from build123d import *

# Parameters (mm, degrees)
BOSS_EXTRUDE1_DEPTH = 5
SKETCH2_R           = 4
CUT_EXTRUDE1_DEPTH  = 5


with BuildPart() as part:
    # Sketch1 → Boss-Extrude1 (new body)
    with BuildSketch(Plane.XY):
        Polygon((-27.36941191, 43.029850731), (-27.36941191, -10.970149254), (-72.36941191, -10.970149254), (-142.36941191, -10.970149254), (-59.112279179, 4.938410019), align=None)
    extrude(amount=BOSS_EXTRUDE1_DEPTH)

    # Sketch2 → Cut-Extrude1 (cut)
    with BuildSketch(Plane.XY.offset(5)):
        with Locations((-37.419438967, -3.470149254)):
            Circle(SKETCH2_R)
        with Locations((-37.419438967, 11.529850746)):
            Circle(SKETCH2_R)
        with Locations((-52.419438967, -4.105668706)):
            Circle(SKETCH2_R)
    extrude(amount=-CUT_EXTRUDE1_DEPTH, mode=Mode.SUBTRACT)


solid = part.part
CAD build for the part. Positions are in the model's coordinates, mm. Coordinates: 2 decimals unless noted, no trailing zeros. Write each loop counter-clockwise with the first axis right and the second up, starting at its lowest first coordinate (ties: lowest second). Pieces come first, ordered by that corner, then holes. Notation, with made-up numbers: (87, 36) - (129, 36) arc R14 cw to (129, 62) - close; hole circle Ø5 at (61.5, 13.5). An arc over 180 degrees is marked (long way). Use a Markdown table: item, result. Add a question column.
Item 1: Band-saw the part on C-C, the plane z = 3.7. Give the cut face in (x, y), and give its area (3 significant figures).
Item 2: Mould opens along X. For faces 1 (the face through (-43.46, 23.72, 2.46)), 2 (the face through (-40.4, 14.2, 2.5)), 3 (the face through (-27.369, 16, 2)) say: pulls with the +X half, pulls with the -X half, needs draft (parallel to the pull), parting line crosses it, or undercut.
Item 3: Band-saw the part on A-A, the plane x = -54. Give the cut face in (y, z).
Item 4: Band-saw the part on D-D, the plane y = 35. Give the cut face in (x, z), and give its area (3 significant figures).
Item 5: Flat gauge pins, fed straight in: pin 1 (9 mm diameter, centred on x = -37.42, y = -3.47, fed in from -Z); pin 2 (1 mm diameter, centred on x = -126.5, z = 1, fed in from +Y); pin 3 (6.5 mm diameter, centred on x = -37.42, y = 11.53, fed in from -Z). Where does each tip first touch, or does it go through?
Item 6: Band-saw the part on B-B, the plane y = 14. Give the cut face in (x, z), and give its area (3 significant figures).
Item 7: Drill centre lines: L1, parallel to X at y = 10, z = 0.45; L2, parallel to Y at x = -40.5, z = 4.4; L3, parallel to X at y = 33.5, z = 3.1. Where is each one in solid material? Low to high. Write a range as from..to.
Numbers:
| question | item | result |
|---|---|---|
| 1 | outline | (-142.37, -10.97) - (-27.37, -10.97) - (-27.37, 43.03) - (-59.11, 4.94) - close; hole circle Ø8 at (-52.42, -4.11); hole circle Ø8 at (-37.42, -3.47); hole circle Ø8 at (-37.42, 11.53) |
| 1 | area | 1,620 mm2 |
| 2 | face 1 | pulls with the -X half |
| 2 | face 2 | undercut |
| 2 | face 3 | pulls with the +X half |
| 3 | outline | (-10.97, 0) - (-7.78, 0) - (-7.78, 5) - (-10.97, 5) - close; (-0.43, 0) - (11.07, 0) - (11.07, 5) - (-0.43, 5) - close |
| 4 | outline | (-34.06, 0) - (-27.37, 0) - (-27.37, 5) - (-34.06, 5) - close |
| 4 | area | 33.5 mm2 |
| 5 | pin 1 | z = 0 |
| 5 | pin 2 | y = -7.84 |
| 5 | pin 3 | through |
| 6 | outline | (-51.56, 0) - (-40.57, 0) - (-40.57, 5) - (-51.56, 5) - close; (-34.27, 0) - (-27.37, 0) - (-27.37, 5) - (-34.27, 5) - close |
| 6 | area | 89.5 mm2 |
| 7 | L1 | -54.89..-41.12, -33.72..-27.37 |
| 7 | L2 | -10.97..-6.02, -0.92..8.98, 14.08..27.27 |
| 7 | L3 | -35.31..-27.37 |
